Work out the finished part from the listing and answer in its coordinate system (mm). A direction names the side the tool comes from. Round coordinates to 2 decimals unless told otherwise and drop trailing zeros. Order: outer loops, then holes, each group sorted by start corner. A loop starts at its lowest first (then second) coordinate and runs counter-clockwise, first axis right, second up.
from build123d import *

# Parameters (mm, degrees)
SKETCH1_R                = 4.7
BOSS_EXTRUDE1_DEPTH      = 19
BOSS_EXTRUDE1_DEPTH_BACK = 19
SKETCH2_R                = 4.7
BOSS_EXTRUDE2_DEPTH      = 19
BOSS_EXTRUDE2_DEPTH_BACK = 19


with BuildPart() as part:
    # Sketch1 → Boss-Extrude1 (new body, two sides)
    with BuildSketch(Plane.XY) as boss_extrude1_sk:
        Circle(SKETCH1_R)
    extrude(amount=BOSS_EXTRUDE1_DEPTH)
    extrude(boss_extrude1_sk.sketch, amount=-BOSS_EXTRUDE1_DEPTH_BACK)

    # Sketch2 → Boss-Extrude2 (add, two sides)
    with BuildSketch(Plane(origin=(0, 0, 0), x_dir=(1, 0, 0), z_dir=(0, 1, 0))) as boss_extrude2_sk:
        Circle(SKETCH2_R)
    extrude(amount=BOSS_EXTRUDE2_DEPTH)
    extrude(boss_extrude2_sk.sketch, amount=-BOSS_EXTRUDE2_DEPTH_BACK)


solid = part.part
Item 1: Find section C-C (y = -3.5). Write down the section's boundary in (x, z).
Item 2: Find the intervals of material crossed by line 1 along Z through (x, y) = (0, 11); line 2 along Y through (x, z) = (-3.75, 17); line 3 along Z through (x, y) = (4, 9.5), in increasing order.
Item 3: Given pin 1 (5 mm diameter, centred on x = 1, z = 7.5, fed in from -Y); pin 2 (1.5 mm diameter, centred on y = -1, z = 5.5, fed in from +X); pin 3 (1.5 mm diameter, centred on y = -9, z = 2, fed in from +X), each flat-ended and moving along its own axis, determine where each tip first touches the part or whether it passes through.
Item 4: Find section D-D (x = -1.5). Write down the section's boundary in (y, z), plus the area to 3 significant figures.
Item 5: Find section B-B (z = 4). Write down the section's boundary in (x, y), plus the area to 3 significant figures.
Item 6: Find section A-A (x = 0.5). Write down the section's boundary in (y, z).
Item 7: A tool of negligible diameter and unlimited length cuts with its end or side. For faces 1 (the face through (-3.7, -11.5, 2.9)), 2 (the face through (-3.7, 11.5, 2.9)), 3 (the face through (-3.7, -2.9, -11.5)), 4 (the face through (-4.695, 0.207, 11.744)), 5 (the face through (0, 0, -19)), from which of +Z, -Z, +X, -X, +Y, -Y can it reach the whole face along a straight path? Write none if from no direction.
Model answer:
1. outline: (-3.14, -19) - (3.14, -19) - (3.14, -3.5) arc R4.7 ccw to (3.14, 3.5) - (3.14, 19) - (-3.14, 19) - (-3.14, 3.5) arc R4.7 ccw to (-3.14, -3.5) - close
2. line 1: z = -4.7 to 4.7
2. line 2: y = -2.83 to 2.83
2. line 3: z = -2.47 to 2.47
3. pin 1: stops at y = -4.7
3. pin 2: stops at x = 4.69
3. pin 3: stops at x = 4.53
4. outline: (-19, -4.45) - (-4.45, -4.45) - (-4.45, -19) - (4.45, -19) - (4.45, -4.45) - (19, -4.45) - (19, 4.45) - (4.45, 4.45) - (4.45, 19) - (-4.45, 19) - (-4.45, 4.45) - (-19, 4.45) - close
4. area: 598 mm2
5. outline: (-2.47, -19) - (2.47, -19) - (2.47, -4) arc R4.7 ccw to (2.47, 4) - (2.47, 19) - (-2.47, 19) - (-2.47, 4) arc R4.7 ccw to (-2.47, -4) - close
5. area: 213 mm2
6. outline: (-19, -4.67) - (-4.67, -4.67) - (-4.67, -19) - (4.67, -19) - (4.67, -4.67) - (19, -4.67) - (19, 4.67) - (4.67, 4.67) - (4.67, 19) - (-4.67, 19) - (-4.67, 4.67) - (-19, 4.67) - close
7. face 1: -Y
7. face 2: +Y
7. face 3: -Z
7. face 4: +Z
7. face 5: -Z, +X, -X, +Y, -Y
